Read the model definition and answer for the solid it produces. Units are mm, in the model's axes. Face numbers are marked on the shaded views. A direction names the side the tool comes from. Coordinates: 2 decimals unless noted, no trailing zeros. Loops run counter-clockwise (first coordinate to the right, second up) from the corner with the lowest first, then second, coordinate; pieces in that order, holes last. Notation, with made-up numbers: M 0,-35 L 56,-35 A19 ccw 56,-31 Z; hole C 45.5,45.25 d8. An arc over 180 degrees is marked long. One line per item, written item: value. Start each with the question number.
1. Determine the mould class of the marked faces 4, 5 and 6 for opening direction Z: +Z half, -Z half, draft (parallel to the pull), parting line (faces both ways), or undercut.
2. The part is cut by section B-B (z = 4.5). Write down the section's boundary in (x, y).
3. For the marked faces 1, 2 and 3, determine the directions among +Z, -Z, +X, -X, +Y, -Y from which every point of the face is accessible in a straight line to the end or side of a thin tool.
4. Consider probe 1 along Y at (x, z) = (-29.05, -45); probe 2 along Y at (x, z) = (-29, 4); probe 3 along Z at (x, y) = (-16, 9.25). Determine where each line is inside the solid, lowest interval first.
5. The part is cut by section C-C (z = -30). Write down the section's boundary in (x, y), then the cut area to 3 significant figures.
6. Flat-ended cylindrical pins translate along their axes: pin 1 (4 mm diameter, centred on x = -35.5, y = 10, fed in from -Z); pin 2 (5 mm diameter, centred on x = -16, y = 3.5, fed in from +Z); pin 3 (7.5 mm diameter, centred on y = 12, z = -43, fed in from -X); pin 4 (3.5 mm diameter, centred on y = 14.8, z = 4.5, fed in from +X). Find the tip coordinate at first contact, or state that the pin passes through.
7. The part is cut by section A-A (y = 14.8). Write down the section's boundary in (x, z), then the cut area to 3 significant figures.
8. The part is cut by section D-D (y = 4.5). Write down the section's boundary in (x, z), then the cut area to 3 significant figures.
```python
from build123d import *

# Parameters (mm, degrees)
BOSS_EXTRUDE1_DEPTH = 20
BOSS_EXTRUDE2_DEPTH = 4
SKETCH3_R           = 2
CUT_EXTRUDE1_DEPTH  = 32.2
SKETCH4_R           = 1.5
CUT_EXTRUDE2_DEPTH  = 2


with BuildPart() as part:
    # Sketch1 → Boss-Extrude1 (new body)
    with BuildSketch(Plane(origin=(0, 0, 0), x_dir=(1, 0, 0), z_dir=(0, 1, 0))):
        Polygon((0, 0), (0, 40.5), (-28, 40.5), (-28, 47.5), (-31.2, 47.5), (-31.2, 40.5), (-38.031373033, 40.5), (-42, 36), (-42, 24), (-41, 23.118082896), (-41, 0), (-31.2, 0), (-31.2, -7), (-28, -7), (-28, 0), align=None)
    extrude(amount=BOSS_EXTRUDE1_DEPTH)

    # Sketch2 → Boss-Extrude2 (add)
    with BuildSketch(Plane.ZY.offset(42)):
        Polygon((-33.464101615, 10), (-31.732050808, 7), (-28.267949192, 7), (-26.535898385, 10), (-28.267949192, 13), (-31.732050808, 13), align=None)
    extrude(amount=BOSS_EXTRUDE2_DEPTH)

    # Sketch3 → Cut-Extrude1 (cut, through all)
    with BuildSketch(Plane.ZY.offset(31.2)):
        with Locations((-45, 5.2)):
            Circle(SKETCH3_R)
        with Locations((-45, 14.8)):
            Circle(SKETCH3_R)
        with Locations((4.5, 14.8)):
            Circle(SKETCH3_R)
        with Locations((4.5, 5.2)):
            Circle(SKETCH3_R)
    extrude(amount=-CUT_EXTRUDE1_DEPTH, mode=Mode.SUBTRACT)

    # Sketch4 → Cut-Extrude2 (cut)
    with BuildSketch(Plane.ZY.offset(46)):
        with Locations((-30, 10)):
            Circle(SKETCH4_R)
    extrude(amount=-CUT_EXTRUDE2_DEPTH, mode=Mode.SUBTRACT)


solid = part.part
```
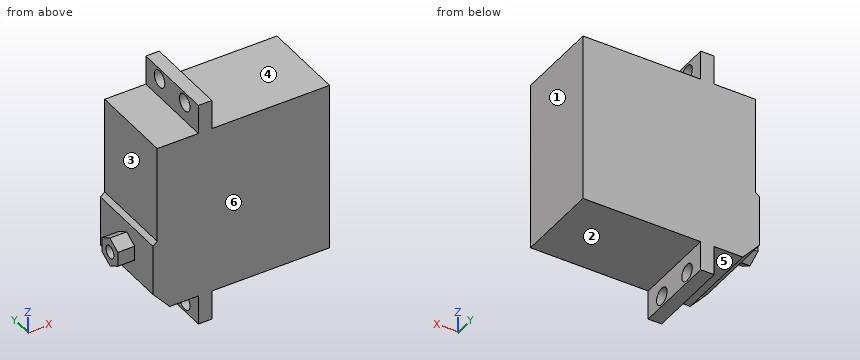
Answer block:
1. face 4: +Z half
1. face 5: -Z half
1. face 6: draft
2. outline: M -31.2,0 L -28,0 L -28,3.2 L -31.2,3.2 Z; M -31.2,7.2 L -28,7.2 L -28,12.8 L -31.2,12.8 Z; M -31.2,16.8 L -28,16.8 L -28,20 L -31.2,20 Z
3. face 1: +Z, -Z, +X, +Y, -Y
3. face 2: -Z, +X, +Y, -Y
3. face 3: +Z, -X, +Y, -Y
4. probe 1: y = 0 to 3.2, 7.2 to 12.8, 16.8 to 20
4. probe 2: y = 0 to 3.26, 7.14 to 12.86, 16.74 to 20
4. probe 3: z = -40.5 to 0
5. outline: M -46,7 L -42,7 L -42,0 L 0,0 L 0,20 L -42,20 L -42,13 L -46,13 L -46,11.5 L -44,11.5 L -44,8.5 L -46,8.5 Z
5. area: 858 mm2
6. pin 1: stops at z = -40.5
6. pin 2: stops at z = 0
6. pin 3: stops at x = -39.13
6. pin 4: passes through
7. outline: M -42,-36 L -38.03,-40.5 L -31.2,-40.5 L -31.2,-43 L -28,-43 L -28,-40.5 L 0,-40.5 L 0,0 L -28,0 L -28,2.5 L -31.2,2.5 L -31.2,0 L -41,0 L -41,-23.12 L -42,-24 Z; M -31.2,-47.5 L -28,-47.5 L -28,-47 L -31.2,-47 Z; M -31.2,6.5 L -28,6.5 L -28,7 L -31.2,7 Z
7. area: 1,690 mm2
8. outline: M -42,-36 L -38.03,-40.5 L -31.2,-40.5 L -31.2,-43.13 L -28,-43.13 L -28,-40.5 L 0,-40.5 L 0,0 L -28,0 L -28,2.63 L -31.2,2.63 L -31.2,0 L -41,0 L -41,-23.12 L -42,-24 Z; M -31.2,-47.5 L -28,-47.5 L -28,-46.87 L -31.2,-46.87 Z; M -31.2,6.37 L -28,6.37 L -28,7 L -31.2,7 Z
8. area: 1,690 mm2
